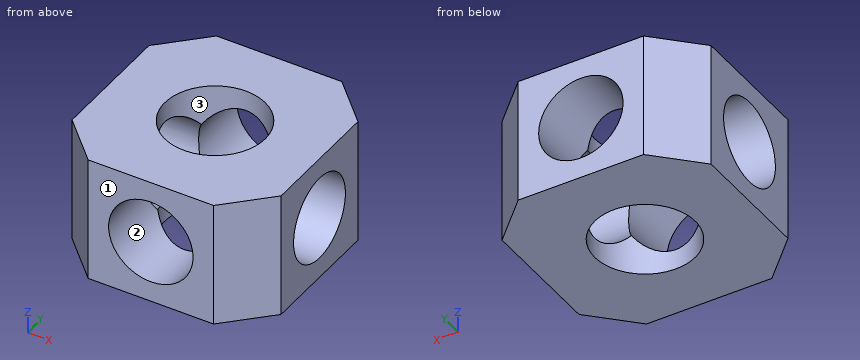
Autodesk Inventor part; units mm, degrees
ref_plane "YZ Plane" through (0, 0, 0) normal (1, 0, 0) x (0, 1, 0)
ref_plane "XZ Plane" through (0, 0, 0) normal (0, 1, 0) x (-1, 0, 0)
ref_plane "XY Plane" through (0, 0, 0) normal (0, 0, 1) x (1, 0, 0)
sketch "Sketch1" plane through (0, 0, 0) normal (0, 0, 1) x (1, 0, 0)
  point P0 (0, 0)
sketch "Sketch2" plane through (0, 0, 0) normal (0, 0, 1) x (1, 0, 0)
  line L0 (0, 0) -> (25, 0)
  line L1 (25, 0) -> (25, 25)
  line L2 (25, 25) -> (0, 25)
  line L3 (0, 25) -> (0, 0)
  dimension "d0" = 25
  dimension "d1" = 25
extrude "Extrusion1" add sketch "Sketch2" along normal blind 15
chamfer "Chamfer1" distance 5 angle 45 4 edges at (25, 25, 7.5) (25, 0, 7.5) (0, 25, 7.5) (0, 0, 7.5)
sketch "Sketch3" plane through (0, 0, 15) normal (0, 0, 1) x (1, 0, 0)
  line L0 (20, 25) -> (5, 25)
  circle A0 centre (12.5, 12.5) radius 6
  line L1 (25, 5) -> (25, 20)
  point P0 (0, 0)
  dimension "d7" = 12
  dimension "d8" = 12.5
  dimension "d9" = 12.5
extrude "Extrusion2" cut sketch "Sketch3" against normal blind 15
sketch "Sketch4" plane through (0, 5, 0) normal (-1, 0, 0) x (0, 0, 1)
  circle A0 centre (7.5, 7.5) radius 5.05
  line L0 (15, 20) -> (0, 20)
  line L1 (15, 15) -> (15, 0)
  point P0 (0, -5)
  dimension "d12" = 10.1
  dimension "d13" = 12.5
  dimension "d14" = 7.5
extrude "Extrusion3" cut sketch "Sketch4" against normal through all
sketch "Sketch5" plane through (5, 25, 0) normal (0, 1, 0) x (1, 0, 0)
  circle A0 centre (7.5, -7.5) radius 5.05
  line L0 (15, 0) -> (0, 0)
  line L1 (-5, 0) -> (-5, -15)
  dimension "d17" = 10.1
  dimension "d18" = 7.5
  dimension "d19" = 12.5
extrude "Extrusion4" cut sketch "Sketch5" against normal through all
properties part number "nut"
Geometry check sheet. Reference: the model listing, model coordinates, mm. Face numbers are marked on the shaded views. Round coordinates to 2 decimals unless told otherwise and drop trailing zeros. Write each loop counter-clockwise with the first axis right and the second up, starting at its lowest first coordinate (ties: lowest second). Pieces come first, ordered by that corner, then holes.
Item 1: Go/stop test with a flat-tipped pin: pin 1 Ø1 at (y, z) = (7.5, 12) entering from -X. Record where the tip stops, or that it passes through.
Determined:
pin 1: stops at x = 0
Item 2: Section check A-A (z = 13.75). Record the boundary of the cut face in (x, y), plus the area to 3 significant figures.
Determined:
outline: (0, 5) - (5, 0) - (20, 0) - (25, 5) - (25, 20) - (20, 25) - (5, 25) - (0, 20) - close; hole circle Ø12 at (12.5, 12.5)
area: 462 mm2
Item 3: Mould release check, pull along Y, two halves, no side actions. Record for the marked faces 1, 2 and 3: +Y half, -Y half, draft (parallel to the pull), parting line (faces both ways), or undercut.
Determined:
face 1: -Y half
face 2: draft
face 3: undercut
Item 4: Material ranges on line 1 along Z through (x, y) = (12.5, 23.75); line 2 along Y through (x, z) = (12.5, 1), recorded low to high.
Determined:
line 1: z = 0 to 2.45, 12.55 to 15
line 2: y = 0 to 6.5, 18.5 to 25
Item 5: Section check B-B (z = 7.5). Record the boundary of the cut face in (x, y), plus the area to 3 significant figures.
Determined:
outline: (0, 5) - (5, 0) - (7.45, 0) - (7.45, 7.45) - (0, 7.45) - close; (0, 17.55) - (7.45, 17.55) - (7.45, 25) - (5, 25) - (0, 20) - close; (17.55, 0) - (20, 0) - (25, 5) - (25, 7.45) - (17.55, 7.45) - close; (17.55, 17.55) - (25, 17.55) - (25, 20) - (20, 25) - (17.55, 25) - close
area: 172 mm2
Item 6: Section check C-C (x = 12.5). Record the boundary of the cut face in (y, z), plus the area to 3 significant figures.
Determined:
outline: (0, 0) - (6.5, 0) - (6.5, 2.45) - (0, 2.45) - close; (0, 12.55) - (6.5, 12.55) - (6.5, 15) - (0, 15) - close; (18.5, 0) - (25, 0) - (25, 2.45) - (18.5, 2.45) - close; (18.5, 12.55) - (25, 12.55) - (25, 15) - (18.5, 15) - close
area: 63.7 mm2
